from build123d import *

# Parameters (mm, degrees)
SKETCH1_R               = 15
BOSS_EXTRUDE1_DEPTH     = 10
CUT_EXTRUDE1_DEPTH      = 189.54707635
CUT_EXTRUDE1_DEPTH_BACK = 189.54707635
SKETCH2_R               = 1.6
SKETCH4_R               = 20
SKETCH4_R_2             = 2.6
CUT_EXTRUDE3_DEPTH      = 189.54707635


with BuildPart() as part:
    # Sketch1 → Boss-Extrude1 (new body)
    with BuildSketch(Plane(origin=(0, 0, 0), x_dir=(1, 0, 0), z_dir=(0, 1, 0))):
        with BuildLine():
            Line((35, 150), (35, -150))
            ThreePointArc((35, -150), (0, -185), (-35, -150))
            Line((-35, -150), (-35, 150))
            ThreePointArc((-35, 150), (0, 185), (35, 150))
        make_face()
        with Locations(Location((0, -150, 0), (0, 0, 270))):
            Circle(SKETCH1_R, mode=Mode.SUBTRACT)
        with Locations(Location((0, 150, 0), (0, 0, 270))):
            Circle(SKETCH1_R, mode=Mode.SUBTRACT)
    extrude(amount=BOSS_EXTRUDE1_DEPTH)

    # Sketch2 → Cut-Extrude1 (cut, two sides: drawn at the far end of the back side and taken through both)
    with BuildSketch(Plane(origin=(0, 10, 0), x_dir=(1, 0, 0), z_dir=(0, 1, 0)).offset(-CUT_EXTRUDE1_DEPTH_BACK)):
        with Locations(Location((-25, 5, 0), (0, 0, 270))):
            Circle(SKETCH2_R)
        with Locations(Location((-25, -5, 0), (0, 0, 270))):
            Circle(SKETCH2_R)
        with Locations(Location((25, -5, 0), (0, 0, 270))):
            Circle(SKETCH2_R)
        with Locations(Location((25, 5, 0), (0, 0, 270))):
            Circle(SKETCH2_R)
        with Locations(Location((25, 95, 0), (0, 0, 270))):
            Circle(SKETCH2_R)
        with Locations(Location((25, 105, 0), (0, 0, 270))):
            Circle(SKETCH2_R)
        with Locations(Location((-25, 105, 0), (0, 0, 270))):
            Circle(SKETCH2_R)
        with Locations(Location((-25, 95, 0), (0, 0, 270))):
            Circle(SKETCH2_R)
        with Locations(Location((-25, -95, 0), (0, 0, 270))):
            Circle(SKETCH2_R)
        with Locations(Location((-25, -105, 0), (0, 0, 270))):
            Circle(SKETCH2_R)
        with Locations(Location((25, -105, 0), (0, 0, 270))):
            Circle(SKETCH2_R)
        with Locations(Location((25, -95, 0), (0, 0, 270))):
            Circle(SKETCH2_R)
    extrude(amount=CUT_EXTRUDE1_DEPTH + CUT_EXTRUDE1_DEPTH_BACK, mode=Mode.SUBTRACT)

    # Sketch4 → Cut-Extrude3 (cut, through all)
    with BuildSketch(Plane.XZ):
        with Locations(Location((0, -50, 0), (0, 0, 270))):
            Circle(SKETCH4_R)
        with Locations(Location((-23.57, -26.43, 0), (0, 0, 270))):
            Circle(SKETCH4_R_2)
        with Locations(Location((23.57, -26.43, 0), (0, 0, 270))):
            Circle(SKETCH4_R_2)
        with Locations(Location((23.57, -73.57, 0), (0, 0, 270))):
            Circle(SKETCH4_R_2)
        with Locations(Location((-23.57, -73.57, 0), (0, 0, 270))):
            Circle(SKETCH4_R_2)
        with BuildLine():
            Line((-25, -82), (25, -82))
            ThreePointArc((25, -82), (28, -85), (25, -88))
            Line((25, -88), (-25, -88))
            ThreePointArc((-25, -88), (-28, -85), (-25, -82))
        make_face()
    cut_extrude3 = extrude(amount=-CUT_EXTRUDE3_DEPTH, mode=Mode.SUBTRACT)

    # Mirror1: Cut-Extrude3 across plane
    add(cut_extrude3.mirror(Plane.XY), mode=Mode.SUBTRACT)


solid = part.part
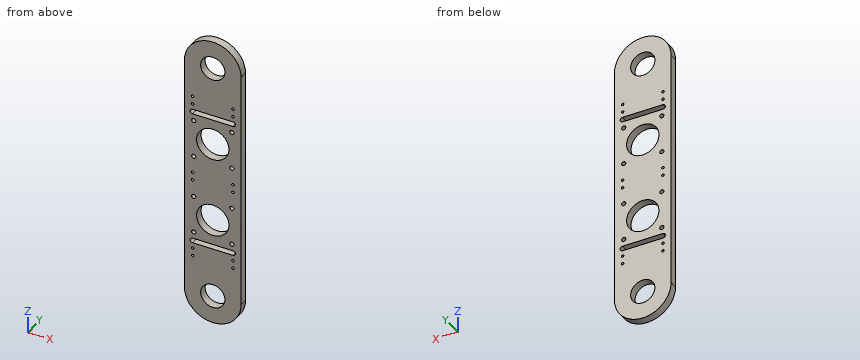
The model under review builds one solid part; all positions refer to its coordinate system, in mm. Give positions to 0.01 mm unless a question says otherwise; leave off trailing zeros. Write each loop counter-clockwise with the first axis right and the second up, starting at its lowest first coordinate (ties: lowest second). Pieces come first, ordered by that corner, then holes.
1. For P1, Ø5, axis at x = 8, y = 2.5, coming from the -Z side; P2, Ø4, axis at x = -23.57, z = -26.43, coming from the -Y side; P3, Ø5, axis at x = 5.5, y = 2, coming from the -Z side; P4, Ø3, axis at x = 7, y = 4.5, coming from the +Z side, all flat-tipped, find the tip position at first contact; note any pin that passes through.
2. Add section A-A, the plane x = 0. Write out the cut boundary in (y, z).
3. Add section C-C, the plane y = 6. Count the separate pieces of the cut face and the enclosed holes in it, plus the area to 3 significant figures.
4. Add section D-D, the plane z = 143. Write out the cut boundary in (x, y).
5. Wall thickness on L1, parallel to X at y = 5.5, z = 26; L2, parallel to X at y = 4.5, z = 26.43; L3, parallel to X at y = 7.5, z = 50: over which ranges is each line inside the solid? List them lowest first.
6. Add section B-B, the plane z = -54.5. Write out the cut boundary in (x, y), plus the area to 3 significant figures.
Worked answers:
1. P1: stops at z = -184.57
1. P2: passes through
1. P3: stops at z = -184.87
1. P4: stops at z = 184.57
2. outline: (0, -185) - (10, -185) - (10, -165) - (0, -165) - close; (0, -135) - (10, -135) - (10, -88) - (0, -88) - close; (0, -82) - (10, -82) - (10, -70) - (0, -70) - close; (0, -30) - (10, -30) - (10, 30) - (0, 30) - close; (0, 70) - (10, 70) - (10, 82) - (0, 82) - close; (0, 88) - (10, 88) - (10, 135) - (0, 135) - close; (0, 165) - (10, 165) - (10, 185) - (0, 185) - close
3. separate pieces: 1
3. enclosed holes: 26
3. area: 20,000 mm2
4. outline: (-35, 0) - (-13.27, 0) - (-13.27, 10) - (-35, 10) - close; (13.27, 0) - (35, 0) - (35, 10) - (13.27, 10) - close
5. L1: x = -35 to -26.13, -21.01 to 21.01, 26.13 to 35
5. L2: x = -35 to -26.17, -20.97 to 20.97, 26.17 to 35
5. L3: x = -35 to -20, 20 to 35
6. outline: (-35, 0) - (-19.49, 0) - (-19.49, 10) - (-35, 10) - close; (19.49, 0) - (35, 0) - (35, 10) - (19.49, 10) - close
6. area: 310 mm2
